Input: dimensioned drawing with shaded views. Units: mm. Origin: part minimum x, y, z. Coordinates: 2 decimals unless noted, no trailing zeros. Order: outer loops, then holes, each group sorted by start corner. A loop starts at its lowest first (then second) coordinate and runs counter-clockwise, first axis right, second up.
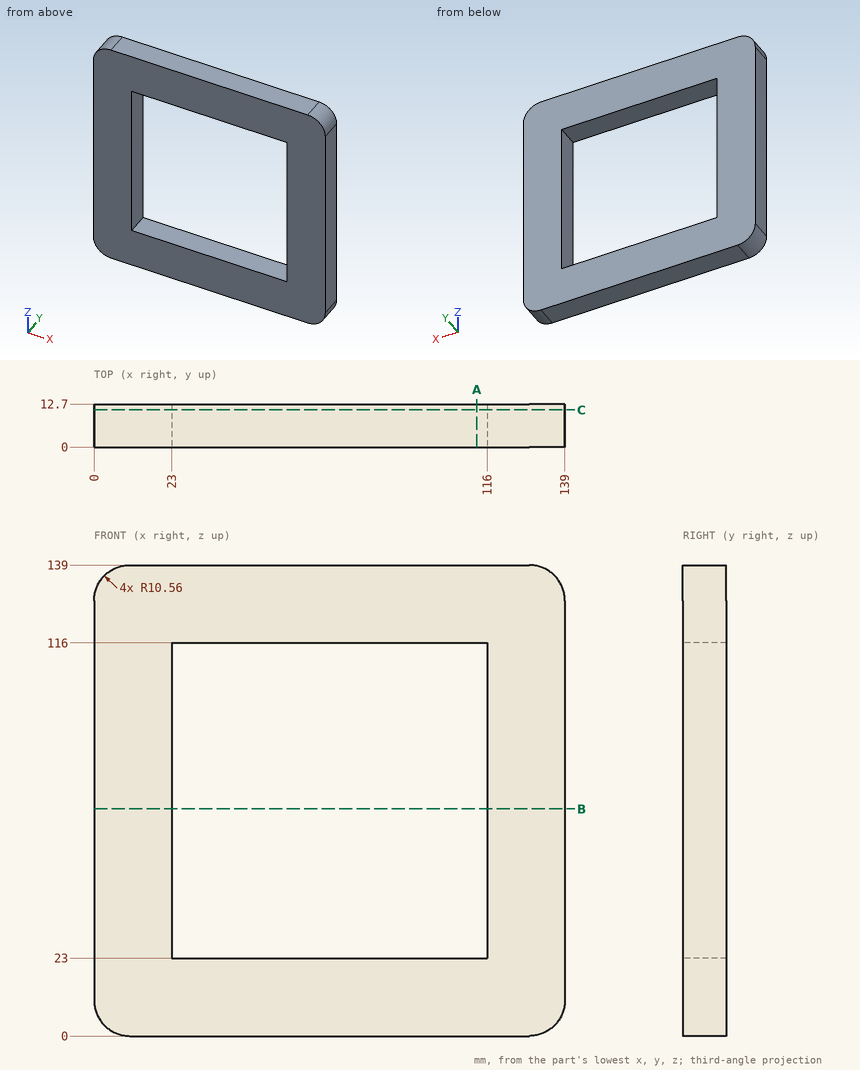
1. Section query C-C on y = 11. Return loops of the section in (x, z), plus the area to 3 significant figures.
Findings:
outline: (0, 10.56) arc R10.56 ccw to (10.56, 0) - (128.44, 0) arc R10.56 ccw to (139, 10.56) - (139, 128.44) arc R10.56 ccw to (128.44, 139) - (10.56, 139) arc R10.56 ccw to (0, 128.44) - close; hole (23, 23) - (116, 23) - (116, 116) - (23, 116) - close
area: 10,600 mm2
2. Section query A-A on x = 113. Return loops of the section in (y, z), plus the area to 3 significant figures.
Findings:
outline: (0, 0) - (12.7, 0) - (12.7, 23) - (0, 23) - close; (0, 116) - (12.7, 116) - (12.7, 139) - (0, 139) - close
area: 584 mm2
3. Pin query (flat end, axial travel): P1, Ø6, axis at x = 25.5, z = 40.5, coming from the +Y side. Return the tip coordinate at first contact, or that it passes through.
Findings:
P1: stops at y = 12.7
4. Section query B-B on z = 67. Return loops of the section in (x, y).
Findings:
outline: (0, 0) - (23, 0) - (23, 12.7) - (0, 12.7) - close; (116, 0) - (139, 0) - (139, 12.7) - (116, 12.7) - close
5. Ray query, line 1 (X direction, y = 9.75, z = 38); line 2 (Z direction, x = 129.5, y = 9). Return the intervals inside material, ascending.
Findings:
line 1: x = 0 to 23, 116 to 139
line 2: z = 0.05 to 138.95
